Check sheet for the drawn part. Datum: minimum x, y, z corner. Units: mm. A direction names the side the tool comes from. Coordinates: 2 decimals unless noted, no trailing zeros. Write each loop counter-clockwise with the first axis right and the second up, starting at its lowest first coordinate (ties: lowest second). Pieces come first, ordered by that corner, then holes. Notation, with made-up numbers: (25, 32) -> (38, 32) arc R26 ccw to (38, 60) -> close; hole circle Ø8 at (3.5, -8). An arc over 180 degrees is marked (long way). Write item = value, one per line. Start each with the question number.
(1) Section check D-D (y = 63). Record the cut outline in (x, z) (1 decimal).
(2) Section check C-C (x = 14). Record the cut outline in (y, z) (1 decimal).
(3) Gauge pin test, flat ends, axial feed: pin 1 Ø8 at (y, z) = (24, 60) entering from -X (1 decimal); pin 2 Ø6 at (x, y) = (27, 47.5) entering from +Z; pin 3 Ø1 at (x, y) = (25.5, 8) entering from -Z. Record the tip position at first contact, or that the pin passes through.
(4) Material ranges on probe 1 along Z at (x, y) = (35, 18); probe 2 along X at (y, z) = (30.5, 26); probe 3 along X at (y, z) = (33, 48.5) (1 decimal), recorded low to high. Write a range as [from, to].
(5) Set-up check for the marked faces 1 and 2: record each of +Z, -Z, +X, -X, +Y, -Y from which the full face is reachable in a straight line by a thin tool's end or side.
(6) Section check B-B (x = 68). Record the cut outline in (y, z) (1 decimal).
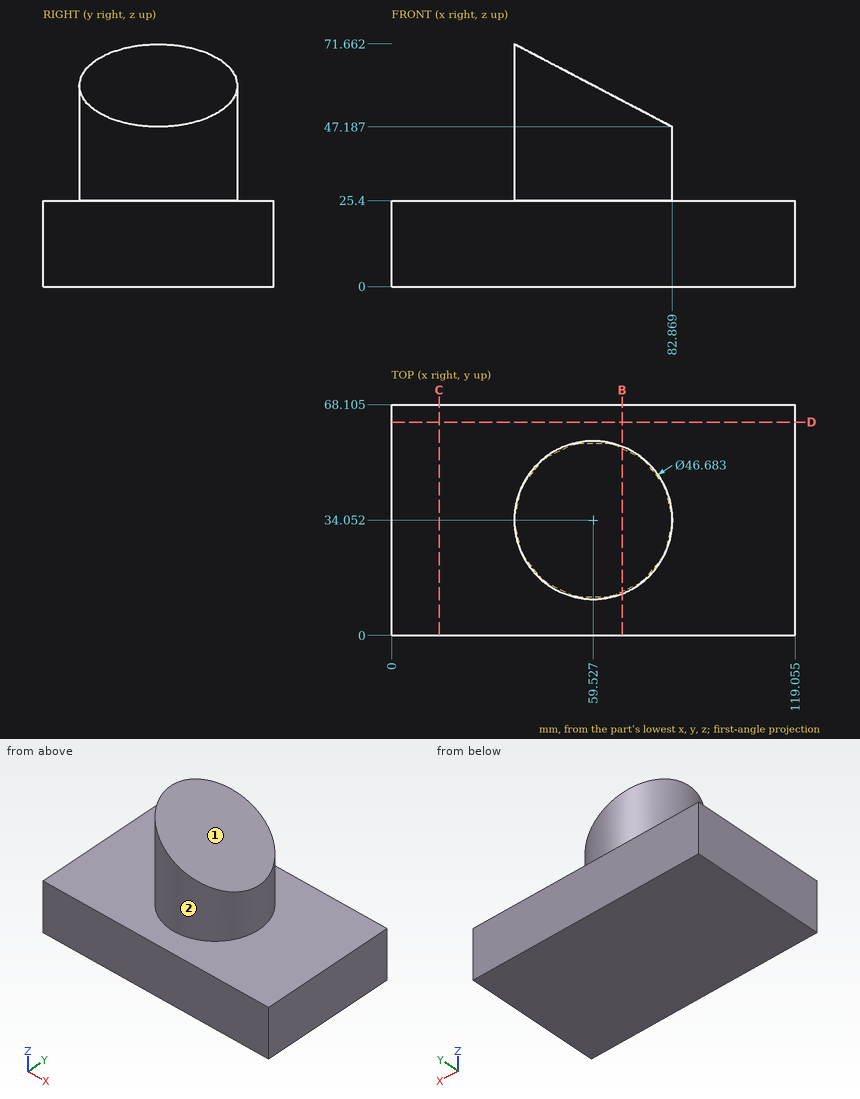
Response:
q1.outline = (0, 0) -> (119.1, 0) -> (119.1, 25.4) -> (0, 25.4) -> close
q2.outline = (0, 0) -> (68.1, 0) -> (68.1, 25.4) -> (0, 25.4) -> close
q3.pin_1 = 37
q3.pin_2 = 25.4
q3.pin_3 = 0
q4.probe_1 = [0, 25.4]
q4.probe_2 = [36.46, 82.6]
q4.probe_3 = [36.2, 80.4]
q5.face_1 = +Z, +X, +Y, -Y
q5.face_2 = +Z
q6.outline = (0, 0) -> (68.1, 0) -> (68.1, 25.4) -> (55.8, 25.4) -> (55.8, 55) -> (12.3, 55) -> (12.3, 25.4) -> (0, 25.4) -> close
